The listing builds one solid part. Answer for the finished solid, in the listing's coordinates (mm). Face numbers are marked on the shaded views. A direction names the side the tool comes from. Coordinates: 2 decimals unless noted, no trailing zeros. Loops run counter-clockwise (first coordinate to the right, second up) from the corner with the lowest first, then second, coordinate; pieces in that order, holes last. Notation, with made-up numbers: (79.5, 36.25) - (122.5, 36.25) arc R15 ccw to (122.5, 55.25) - close; hole circle Ø1 at (-7.5, -10). An arc over 180 degrees is marked (long way). Return JSON: item names as keys, results as strings. Group by question number.
1. Each of these flat-tipped pins is pushed along its axis until it touches: P1, Ø4, axis at y = 88.5, z = -4.5, coming from the +X side; P2, Ø2, axis at y = 107, z = 2.5, coming from the -X side; P3, Ø1.5, axis at x = 11, y = 37, coming from the -Z side; P4, Ø4.5, axis at x = 7.5, y = 97, coming from the +Z side. Where does it stop, or does it pass through?
2. Section B-B (z = 7.75) is taken. Write down the section's boundary in (x, y).
3. Which of the six approach directions +Z, -Z, +X, -X, +Y, -Y give full straight-line access (tool end or side, diameter ignored) to the marked faces 1, 2 and 3?
4. The mould has two halves that part along X. Classify the marked faces 4, 5, 6 and 7: pulls with the +X half, pulls with the -X half, needs draft (parallel to the pull), parting line crosses it, or undercut.
5. Section C-C (y = 30) is taken. Write down the section's boundary in (x, z), and give its area (3 significant figures).
6. Find the intervals of material crossed by line 1 along Y through (x, z) = (7.5, 7); line 2 along Y through (x, z) = (7.5, -6.3); line 3 along X through (y, z) = (6, 7.5), in increasing order.
7. Section A-A (x = 7.5) is taken. Write down the section's boundary in (y, z), and give its area (3 significant figures).
8. Section D-D (y = 70.5) is taken. Write down the section's boundary in (x, z).
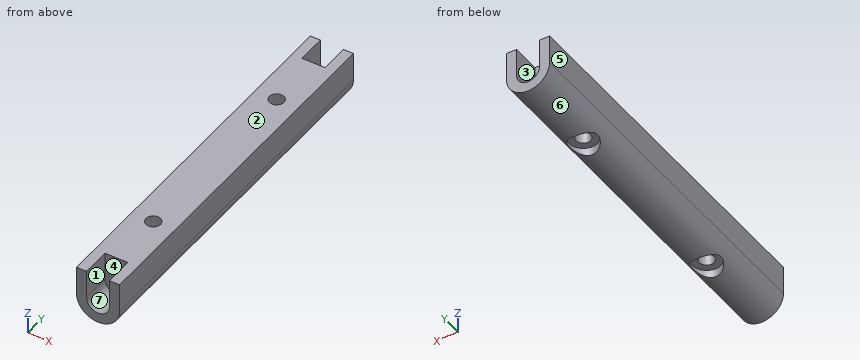
```python
from build123d import *

# Parameters (mm, degrees)
EXTRUDE_1_DEPTH     = 127
SKETCH_6_R          = 2.55
CUT_EXTRUDE_1_DEPTH = 14.5
SKETCH_7_R          = 5
CUT_EXTRUDE_2_DEPTH = 14.5
CUT_EXTRUDE_3_DEPTH = 10
SKETCH_9_R          = 2.55
CUT_EXTRUDE_4_DEPTH = 14.5
SKETCH_10_R         = 5
CUT_EXTRUDE_5_DEPTH = 14.5
CUT_EXTRUDE_START   = -10
CUT_EXTRUDE_6_DEPTH = 10


with BuildPart() as part:
    # Эскиз2 → Бобышка-Вытянуть1 (new body)
    with BuildSketch(Plane(origin=(0, 0, 0), x_dir=(1, 0, 0), z_dir=(0, 1, 0))):
        with BuildLine():
            Line((0, 0), (0, -10))
            Line((0, -10), (15, -10))
            Line((15, -10), (15, 0))
            ThreePointArc((15, 0), (7.5, 7.5), (0, 0))
        make_face()
    extrude(amount=EXTRUDE_1_DEPTH)

    # Эскиз6 → Вырез-Вытянуть1 (cut)
    with BuildSketch(Plane.XY.offset(10)):
        with Locations((7.5, 30)):
            Circle(SKETCH_6_R)
    extrude(amount=-CUT_EXTRUDE_1_DEPTH, mode=Mode.SUBTRACT)

    # Эскиз7 → Вырез-Вытянуть2 (cut)
    with BuildSketch(Plane.XY.offset(-4.5)):
        with Locations((7.5, 30)):
            Circle(SKETCH_7_R)
    extrude(amount=-CUT_EXTRUDE_2_DEPTH, mode=Mode.SUBTRACT)

    # Эскиз8 → Вырез-Вытянуть3 (cut)
    with BuildSketch(Plane.XZ):
        with BuildLine():
            Line((11.5, 0), (11.5, 10))
            Line((11.5, 10), (3.5, 10))
            Line((3.5, 10), (3.5, 0))
            ThreePointArc((3.5, 0), (7.5, -4), (11.5, 0))
        make_face()
    extrude(amount=-CUT_EXTRUDE_3_DEPTH, mode=Mode.SUBTRACT)

    # Эскиз9 → Вырез-Вытянуть4 (cut)
    with BuildSketch(Plane.XY.offset(10)):
        with Locations((7.5, 97)):
            Circle(SKETCH_9_R)
    extrude(amount=-CUT_EXTRUDE_4_DEPTH, mode=Mode.SUBTRACT)

    # Эскиз10 → Вырез-Вытянуть5 (cut)
    with BuildSketch(Plane.XY.offset(-4.5)):
        with Locations((7.5, 97)):
            Circle(SKETCH_10_R)
    extrude(amount=-CUT_EXTRUDE_5_DEPTH, mode=Mode.SUBTRACT)

    # Эскиз11 → Вырез-Вытянуть6 (cut)
    with BuildSketch(Plane(origin=(0, 127, 0), x_dir=(1, 0, 0), z_dir=(0, 1, 0)).offset(CUT_EXTRUDE_START)):
        with BuildLine():
            Line((11.5, 0), (11.5, -10))
            Line((11.5, -10), (3.5, -10))
            Line((3.5, -10), (3.5, 0))
            ThreePointArc((3.5, 0), (7.5, 4), (11.5, 0))
        make_face()
    extrude(amount=CUT_EXTRUDE_6_DEPTH, mode=Mode.SUBTRACT)


solid = part.part
```
The answers:
{
 "1": {"P1": "stops at x = 14.57", "P2": "stops at x = 0", "P3": "stops at z = -6.98", "P4": "passes through"},
 "2": {"outline": "(0, 0) - (3.5, 0) - (3.5, 10) - (11.5, 10) - (11.5, 0) - (15, 0) - (15, 127) - (11.5, 127) - (11.5, 117) - (3.5, 117) - (3.5, 127) - (0, 127) - close; hole circle Ø5.1 at (7.5, 30); hole circle Ø5.1 at (7.5, 97)"},
 "3": {"face 1": "+Z, -Y", "face 2": "+Z, +X, -X, +Y, -Y", "face 3": "+Z, +Y"},
 "4": {"face 4": "undercut", "face 5": "pulls with the -X half", "face 6": "parting line crosses it", "face 7": "undercut"},
 "5": {"outline": "(0, 0) arc R7.5 ccw to (2.5, -5.59) - (2.5, -4.5) - (4.95, -4.5) - (4.95, 10) - (0, 10) - close; (10.05, -4.5) - (12.5, -4.5) - (12.5, -5.59) arc R7.5 ccw to (15, 0) - (15, 10) - (10.05, 10) - close", "area": "140 mm2"},
 "6": {"line 1": "y = 10 to 27.45, 32.55 to 94.45, 99.55 to 117", "line 2": "y = 0 to 25, 35 to 92, 102 to 127", "line 3": "x = 0 to 3.5, 11.5 to 15"},
 "7": {"outline": "(0, -7.5) - (25, -7.5) - (25, -4.5) - (27.45, -4.5) - (27.45, 10) - (10, 10) - (10, -4) - (0, -4) - close; (32.55, -4.5) - (35, -4.5) - (35, -7.5) - (92, -7.5) - (92, -4.5) - (94.45, -4.5) - (94.45, 10) - (32.55, 10) - close; (99.55, -4.5) - (102, -4.5) - (102, -7.5) - (127, -7.5) - (127, -4) - (117, -4) - (117, 10) - (99.55, 10) - close", "area": "1,730 mm2"},
 "8": {"outline": "(0, 0) arc R7.5 ccw to (15, 0) - (15, 10) - (0, 10) - close"}
}
